Can you work these out from the drawing? Everything is in mm from the part's minimum corner. A direction names the side the tool comes from. Round coordinates to 2 decimals unless told otherwise and drop trailing zeros. Loops run counter-clockwise (first coordinate to the right, second up) from the corner with the lowest first, then second, coordinate; pieces in that order, holes last. Notation, with made-up numbers: (4.25, 13.25) -> (53.25, 13.25) arc R27 ccw to (53.25, 46.25) -> close; hole circle Ø10 at (-2, -34). An arc over 180 degrees is marked (long way). One line per item, written item: value.
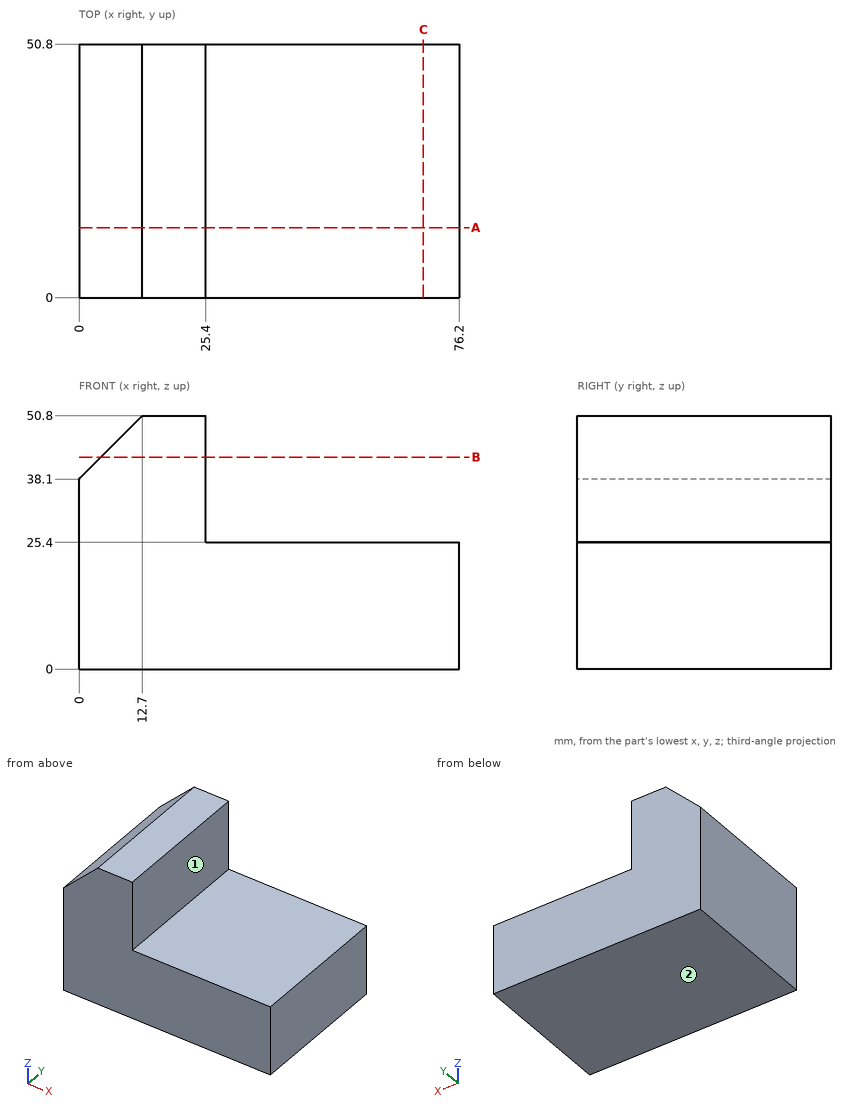
(1) On a 3-axis mill with a long thin cutter (end or side, diameter ignored), from which of +Z, -Z, +X, -X, +Y, -Y can I reach the whole of each face in a straight line? I mean the marked faces 1 and 2. Say none if no direction works.
Results below:
face 1: +Z, +X, +Y, -Y
face 2: -Z, +X, -X, +Y, -Y
(2) Imagine slicing it at A-A on y = 14. Write out the boundary of the cut face in (x, z).
Results below:
outline: (0, 0) -> (76.2, 0) -> (76.2, 25.4) -> (25.4, 25.4) -> (25.4, 50.8) -> (12.7, 50.8) -> (0, 38.1) -> close
(3) Imagine slicing it at C-C on x = 69. Write out the boundary of the cut face in (y, z).
Results below:
outline: (0, 0) -> (50.8, 0) -> (50.8, 25.4) -> (0, 25.4) -> close
(4) Imagine slicing it at B-B on z = 42.5. Write out the boundary of the cut face in (x, y).
Results below:
outline: (4.4, 0) -> (25.4, 0) -> (25.4, 50.8) -> (4.4, 50.8) -> close
(5) For pin 1 Ø1 at (x, y) = (60.5, 41) entering from +Z; pin 2 Ø1.5 at (y, z) = (23, 42.5) entering from +X; pin 3 Ø1.5 at (y, z) = (20, 42.5) entering from -X, each with a flat end and sliding along its axis, tell me the tip position at first contact or that it passes through.
Results below:
pin 1: stops at z = 25.4
pin 2: stops at x = 25.4
pin 3: stops at x = 3.65
(6) Please list where these lines run through material, in increasing order: L1, parallel to Z at x = 44.5, y = 24; L2, parallel to X at y = 42.5, z = 44.5.
Results below:
L1: z = 0 to 25.4
L2: x = 6.4 to 25.4
